from build123d import *

# Parameters (mm, degrees)
F2_R = 6.34999


# Not quite as in the source:
# - a fillet or chamfer is up to 0.001 mm smaller than in the source, because OpenCascade refuses the exact size


with BuildPart() as f1:
    # F0 (on Front) → F1 (revolve)
    with BuildSketch(Plane.XZ):
        Polygon((3.9624, -4.7625), (0, -4.7625), (0, -17.4625), (113.5126, -17.4625), (113.5126, -11.1125), (3.9624, -11.1125), align=None)
    revolve(axis=Axis((63.5, 0, 0), (1, 0, 0)))

    # F2 (radius 6.35 in the source; OpenCascade refuses exactly that, so slightly less here)
    f2_edges = [f1.edges().sort_by_distance(p)[0] for p in [
        (0, 0, 17.4625),
        (113.5126, 0, 17.4625),
    ]]
    fillet(f2_edges, radius=F2_R)


solid = f1.part
Check sheet for the modelled part. Datum: model origin and axes. Units: mm. A direction names the side the tool comes from. Give positions to 0.01 mm unless a question says otherwise; leave off trailing zeros. Write each loop counter-clockwise with the first axis right and the second up, starting at its lowest first coordinate (ties: lowest second). Pieces come first, ordered by that corner, then holes. Notation, with made-up numbers: (37.5, 62) -> (71.5, 62) arc R16 ccw to (71.5, 85) -> close; hole circle Ø2 at (-14, 68). An arc over 180 degrees is marked (long way). Write item = value, one per line.
Item 1: Gauge pin test, flat ends, axial feed: pin 1 (12 mm diameter, centred on x = 90.5, y = -10, fed in from +Z); pin 2 (1 mm diameter, centred on x = 32.5, z = 14, fed in from -Y); pin 3 (6 mm diameter, centred on x = 100, z = 5, fed in from +Y). Record the tip position at first contact, or that the pin passes through.
Output:
pin_1 = 17
pin_2 = -11.08
pin_3 = 17.35
Item 2: Scan lines: probe 1 along Y at (x, z) = (76, 0); probe 2 along X at (y, z) = (2, -4.5); probe 3 along Z at (x, y) = (29, 7). Record each from-to range of solid material in increasing order. Write a range as from..to.
Output:
probe_1 = -17.46..-11.11, 11.11..17.46
probe_2 = 0..3.96
probe_3 = -16..-8.63, 8.63..16
Item 3: Release check for a two-part mould opening along Z. For faces 3 (the flat face through (3.962, -5, 0)), 4 (the flat face through (0, -5, 0)), 5 (the cylindrical face through (57.462, -10.626, 13.858)) record: +Z half, -Z half, draft (parallel to the pull), parting line (faces both ways), or undercut.
Output:
face_3 = undercut
face_4 = draft
face_5 = parting line
Item 4: Tool access check on faces 1 (the cylindrical face through (57.97, 3.34, -10.6)), 2 (the cylindrical face through (1.95, -2.9, 3.78)). Record the directions out of +Z, -Z, +X, -X, +Y, -Y that give a thin tool (end or side, any length) a straight path to the whole face; none if there is none.
Output:
face_1 = +X
face_2 = +X, -X
Item 5: Sectioned sample at C-C on x = 73. Record the boundary of the cut face in (y, z) (1 decimal), and give its area (3 significant figures).
Output:
outline = circle Ø34.9 at (0, 0); hole circle Ø22.2 at (0, 0)
area = 570 mm^2
